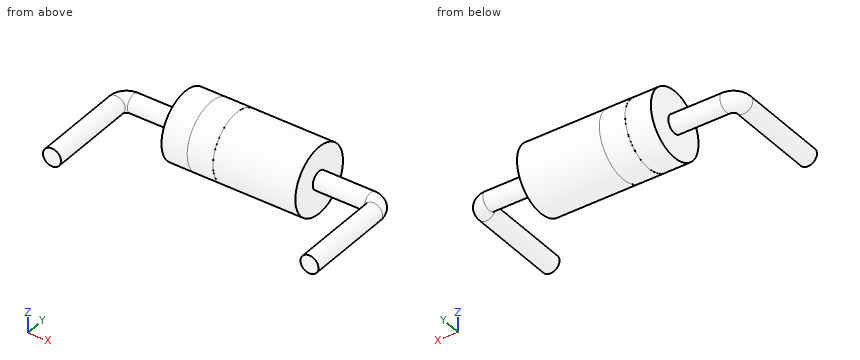
from build123d import *

# Parameters (mm, degrees)
SKIZZE1_R                       = 1.3
AUFSATZ_LINEAR_AUSTRAGEN1_DEPTH = 5.2
SKIZZE4_R                       = 1.302
AUFSATZ_LINEAR_AUSTRAGEN2_DEPTH = 1
SKIZZE10_R                      = 0.35
SKIZZE12_R                      = 0.35


with BuildPart() as part:
    # Skizze1 → Aufsatz-Linear austragen1 (new body)
    with BuildSketch(Plane(origin=(0, 0, 0), x_dir=(0, 0, -1), z_dir=(1, 0, 0))):
        Circle(SKIZZE1_R)
    extrude(amount=AUFSATZ_LINEAR_AUSTRAGEN1_DEPTH)

    # Skizze4 → Aufsatz-Linear austragen2 (add)
    with BuildSketch(Plane.ZY.offset(-2)):
        Circle(SKIZZE4_R)
    extrude(amount=AUFSATZ_LINEAR_AUSTRAGEN2_DEPTH)

    # Austragung3: sweep along a path in Skizze11
    with BuildLine(Plane.XY) as austragung3_path:
        Line((5.2, 0), (7.2, 0))
        ThreePointArc((7.2, 0), (7.482842712, -0.117157288), (7.6, -0.4))
        Line((7.6, -0.4), (7.6, -3.9))
    # Skizze10 → Austragung3 (sweep)
    with BuildSketch(Plane(origin=(5.2, 0, 0), x_dir=(0, 0, -1), z_dir=(1, 0, 0))):
        Circle(SKIZZE10_R)
    sweep(path=austragung3_path.line)

    # Austragung4: sweep along a path in Skizze13
    with BuildLine(Plane.XY) as austragung4_path:
        Line((0, 0), (-2, 0))
        ThreePointArc((-2, 0), (-2.282842712, -0.117157288), (-2.4, -0.4))
        Line((-2.4, -0.4), (-2.4, -3.9))
    # Skizze12 → Austragung4 (sweep)
    with BuildSketch(Plane.ZY):
        Circle(SKIZZE12_R)
    sweep(path=austragung4_path.line)


solid = part.part
Here's how the part is built. I have some questions about the finished solid (model axes, mm). Coordinates: 2 decimals unless noted, no trailing zeros. Loops run counter-clockwise (first coordinate to the right, second up) from the corner with the lowest first, then second, coordinate; pieces in that order, holes last.
1. Imagine slicing it at C-C, the plane x = 3. Please give me the cut outline in (y, z), and give its area (3 significant figures).
2. I need wall thicknesses on L1, parallel to X at y = -0.9, z = 0.45; L2, parallel to X at y = -0.5, z = -0.1; L3, parallel to Y at x = 3.5, z = 0.55. Which ranges of each line are inside material? Lowest first, please.
3. For P1, Ø1.5, axis at x = -0.5, z = 0, coming from the +Y side; P2, Ø0.8, axis at y = 0, z = -0.5, coming from the +X side, each with a flat end and sliding along its axis, tell me the tip position at first contact or that it passes through.
4. Imagine slicing it at B-B, the plane y = -2.55. Please give me the cut outline in (x, z).
Taken from the geometry:
1. outline: circle Ø2.6 at (0, 0)
1. area: 5.31 mm2
2. L1: x = 0 to 5.2
2. L2: x = -2.74 to -2.06, 0 to 5.2, 7.26 to 7.94
2. L3: y = -1.18 to 1.18
3. P1: stops at y = 1.3
3. P2: stops at x = 7.89
4. outline: circle Ø0.7 at (-2.4, 0); circle Ø0.7 at (7.6, 0)
